Source: CAD feature listing. Evaluate the final solid. Frame: model axes, mm. Face numbers are marked on the shaded views. A direction names the side the tool comes from. Coordinates: 2 decimals unless noted, no trailing zeros. Order: outer loops, then holes, each group sorted by start corner. A loop starts at its lowest first (then second) coordinate and runs counter-clockwise, first axis right, second up.
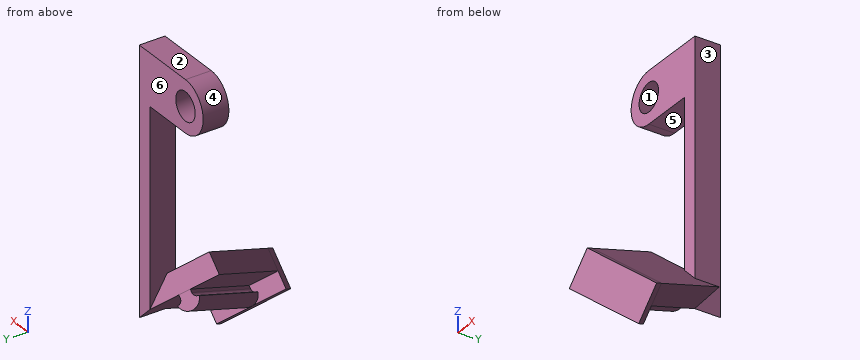
Autodesk Inventor part; units mm, degrees
ref_plane "YZ Plane" through (0, 0, 0) normal (1, 0, 0) x (0, 1, 0)
ref_plane "XZ Plane" through (0, 0, 0) normal (0, 1, 0) x (-1, 0, 0)
ref_plane "XY Plane" through (0, 0, 0) normal (0, 0, 1) x (1, 0, 0)
sketch "Sketch2" plane through (0, 0, 0) normal (0, 1, 0) x (-1, 0, 0)
  circle A0 centre (13.1, 80.1) radius 2.75
  circle A1 centre (80.1, 13.1) radius 2.75 construction
  line L0 (13.1, 80.1) -> (13.1, 13.1)
  line L1 (13.1, 13.1) -> (80.1, 13.1)
  line L2 (3, 37.224) -> (37.224, 3)
  line L3 (3, 37.224) -> (51.4, 37.224) construction
  circle A2 centre (80.1, 13.1) radius 2.75
  line L4 (3.1, 112.1) -> (3.1, 79.1)
  line L5 (79.1, 3.1) -> (112.1, 3.1)
  circle A3 centre (13.1, 80.1) radius 5
  line L6 (13.1, 75.1) -> (3, 75.1)
  line L7 (3, 75.1) -> (3, 3)
  line L8 (13.1, 85.1) -> (0, 85.1)
  line L9 (0, 85.1) -> (0, 0)
  circle A4 centre (80.1, 13.1) radius 5
  line L10 (85.1, 13.1) -> (85.1, 0)
  line L11 (75.1, 13.1) -> (75.1, 3)
  line L12 (75.1, 3) -> (3, 3)
  line L13 (85.1, 0) -> (0, 0)
  line L14 (3, 37.224) -> (-4.0711, 30.1529)
  line L15 (3, 37.224) -> (13, 37.224) construction
  point P0 (0, 0)
  point P1 (0, 34.224)
  dimension "d11" = 48.4
  dimension "d12" = 45
  dimension "d13" = 10
  dimension "d14" = 10.1
  dimension "d15" = 13.1
  dimension "d16" = 3
  dimension "d17" = 10
  dimension "d18" = 13.1
  dimension "d19" = 10.1
  dimension "d20" = 10
  dimension "d21" = 135
extrude "Extrusion2" add sketch "Sketch2" along normal blind 5 contours L6 L7 L14 L9 L8 A3 | A3
sketch "Sketch4" plane through (-3, 0, 37.224) normal (-0.7071068, 0, -0.7071068) x (-0.7071068, 0, 0.7071068)
  line L0 (0, 0) -> (0, 5)
  line L1 (0, 5) -> (-16.134, -14.2277)
  line L2 (0, 5) -> (25.1, 5) construction
  line L3 (-5.9456, -22.7768) -> (10.1884, -3.5491)
  line L4 (10.1884, -3.5491) -> (0, 5)
  line L5 (-5.9456, -22.7768) -> (-16.134, -14.2277)
  point P0 (-28.4426, 0)
  dimension "d33" = 130
  dimension "d34" = 25.1
  dimension "d35" = 13.3
  dimension "d37" = 25.1
extrude "Extrusion3" add sketch "Sketch4" against normal blind 4
sketch "Sketch6" plane through (0, -0.0562, 34.224) normal (-0.7071068, 0, -0.7071068) x (-0.7071068, 0, 0.7071068)
  line L0 (0, 5.0562) -> (4.2426, 5.0562)
  line L1 (0, 0.0562) -> (0, 5.0562)
  line L2 (0.0471, 0.0562) -> (-11.8913, -14.1715)
  line L3 (-11.8913, -14.1715) -> (-1.7029, -22.7206)
  line L4 (-1.7029, -22.7206) -> (14.431, -3.4929)
  line L5 (14.431, -3.4929) -> (4.2426, 5.0562)
  circle A0 centre (6.1229, -3.0486) radius 2.6
  line L6 (4.6432, 4.72) -> (14.755, -3.7647)
  circle A1 centre (-1.5906, -12.2411) radius 2.6
  line L7 (0, 0.0562) -> (0.0471, 0.0562)
  line L8 (14.431, -3.4929) -> (4.2426, 5.0562)
  line L9 (-6.7971, -18.4461) -> (10.7436, 2.4582)
  point P0 (-24.2, 0.0562)
  dimension "d38" = 5.2
  dimension "d39" = 5
  dimension "d40" = 12
extrude "Extrusion5" [suppressed]
fillet "Fillet1" [suppressed]
sketch "Sketch9" plane through (-0.1716, 0, 40.0524) normal (0.7071068, 0, 0.7071068) x (0.7071068, 0, -0.7071068)
  line L0 (4.1955, 0) -> (16.134, -14.2277)
  line L1 (16.134, -14.2277) -> (6.4922, -2.737)
  line L2 (6.4922, -2.737) -> (8.7903, -0.8087)
  line L3 (8.7903, -0.8087) -> (18.4321, -12.2994)
  line L4 (18.4321, -12.2994) -> (16.134, -14.2277)
  line L5 (5.9456, -22.7768) -> (16.134, -14.2277)
  line L6 (11.0398, -18.5023) -> (9.8066, -17.0326)
  line L7 (5.9456, -22.7768) -> (-3.6962, -11.2861)
  line L8 (-5.9944, -13.2145) -> (3.6474, -24.7052)
  line L9 (-3.6962, -11.2861) -> (-5.9944, -13.2145)
  line L10 (3.6474, -24.7052) -> (5.9456, -22.7768)
  point P0 (28.4426, 0)
  point P1 (4.6202, -0.5061)
  dimension "d46" = 15
  dimension "d47" = 3
extrude "Extrusion6" [suppressed]
sketch "Sketch10" plane through (8.4084, -14.2277, 25.8155) normal (0.4545195, -0.7660444, -0.4545195) x (0.7071068, 0, 0.7071068)
  line L0 (0, 0) -> (0, 13.3)
  line L1 (0, 0) -> (4, 0)
  line L2 (4, 13.3) -> (4, 0)
  line L3 (0, 13.3) -> (4, 13.3)
  line L4 (-0.6, 8.15) -> (0, 8.15)
  line L5 (0, -1.85) -> (0, 5.15)
  line L6 (0, 5.15) -> (-0.6, 5.15)
  arc A0 (-0.6, 5.15) -> (-1.099, 4.6815) centre (-0.6, 4.65) ccw
  arc A1 (-1.7225, 4.2287) -> (-1.099, 4.6815) centre (-1.598, 4.713) ccw
  arc A2 (-1.7225, 9.0713) -> (-1.7225, 4.2287) centre (-1.1, 6.65) ccw
  arc A3 (-1.099, 8.6185) -> (-1.7225, 9.0713) centre (-1.598, 8.587) ccw
  arc A4 (-1.099, 8.6185) -> (-0.6, 8.15) centre (-0.6, 8.65) ccw
  line L7 (0, 0) -> (0, 13.3)
  line L8 (0.6, 5.35) -> (-0.6, 5.35)
  arc A5 (-0.6, 5.35) -> (-1.2986, 4.6941) centre (-0.6, 4.65) ccw
  arc A6 (-1.6727, 4.4224) -> (-1.2986, 4.6941) centre (-1.598, 4.713) ccw
  arc A7 (-1.6727, 8.8776) -> (-1.6727, 4.4224) centre (-1.1, 6.65) ccw
  arc A8 (-1.2986, 8.6059) -> (-1.6727, 8.8776) centre (-1.598, 8.587) ccw
  arc A9 (-1.2986, 8.6059) -> (-0.6, 7.95) centre (-0.6, 8.65) ccw
  line L9 (-0.6, 7.95) -> (0.6, 7.95)
  line L10 (0.3, -1.85) -> (0.3, 5.45)
  line L11 (0.3, 5.45) -> (-0.6, 5.45)
  arc A10 (-0.6, 5.45) -> (-1.3984, 4.7004) centre (-0.6, 4.65) ccw
  arc A11 (-1.6478, 4.5193) -> (-1.3984, 4.7004) centre (-1.598, 4.713) ccw
  arc A12 (-1.6478, 8.7807) -> (-1.6478, 4.5193) centre (-1.1, 6.65) ccw
  arc A13 (-1.3984, 8.5996) -> (-1.6478, 8.7807) centre (-1.598, 8.587) ccw
  arc A14 (-1.3984, 8.5996) -> (-0.6, 7.85) centre (-0.6, 8.65) ccw
  line L12 (-0.6, 7.85) -> (0.4, 7.85)
  line L13 (0.4, -1.85) -> (0.4, 5.55)
  line L14 (0.4, 5.55) -> (-0.6, 5.55)
  arc A15 (-0.6, 5.55) -> (-1.4982, 4.7067) centre (-0.6, 4.65) ccw
  arc A16 (-1.6229, 4.6161) -> (-1.4982, 4.7067) centre (-1.598, 4.713) ccw
  arc A17 (-1.6229, 8.6839) -> (-1.6229, 4.6161) centre (-1.1, 6.65) ccw
  arc A18 (-1.4982, 8.5933) -> (-1.6229, 8.6839) centre (-1.598, 8.587) ccw
  arc A19 (-1.4982, 8.5933) -> (-0.6, 7.75) centre (-0.6, 8.65) ccw
  line L15 (-0.6, 7.75) -> (0.4, 7.75)
  point P0 (-24.2, -18.5744)
  point P1 (-11.4165, -11.1867)
  point P2 (0, 6.65)
  point P3 (0, 6.65)
  point P4 (0, 5.35)
  point P5 (0, 7.95)
  point P6 (0, 5.45)
  point P7 (0, 7.85)
  point P8 (0, 5.55)
  point P9 (0, 7.75)
  dimension "d64" = 2.5
  dimension "d65" = 0.6
  dimension "d66" = 1.1
  dimension "d67" = 0.2
  dimension "d68" = 0.3
  dimension "d69" = 0.4
extrude "Extrusion7" add sketch "Sketch10" against normal up to surface (25.1 mm away) contours L14 A15 A16 A17 A18 A19 L15 L0
sketch "Sketch11" plane through (11.2369, -14.2277, 28.644) normal (0.4545195, -0.7660444, -0.4545195) x (0.7071068, 0, 0.7071068)
  line L0 (-4, 0) -> (-4, 5.55)
  line L1 (-4, 0) -> (0, 0)
  line L2 (0, 13.3) -> (0, 0)
  line L3 (-4, 13.3) -> (0, 13.3)
  line L4 (0, 0) -> (0, 13.3)
  line L5 (0, 0) -> (-7.3, 0)
  line L6 (-7.7, 13.3) -> (0, 13.3)
  line L7 (0, 13.3) -> (0, 0)
  line L8 (-4, 7.75) -> (-4, 13.3)
  line L9 (-4, 7.75) -> (-4.6, 7.75)
  arc A0 (-5.4982, 8.5933) -> (-4.6, 7.75) centre (-4.6, 8.65) ccw
  arc A1 (-5.4982, 8.5933) -> (-5.6229, 8.6839) centre (-5.598, 8.587) ccw
  arc A2 (-5.6229, 8.6839) -> (-5.6229, 4.6161) centre (-5.1, 6.65) ccw
  arc A3 (-5.6229, 4.6161) -> (-5.4982, 4.7067) centre (-5.598, 4.713) ccw
  arc A4 (-4.6, 5.55) -> (-5.4982, 4.7067) centre (-4.6, 4.65) ccw
  line L10 (-4.6, 5.55) -> (-4, 5.55)
  line L11 (-7.2, 13.3) -> (-7.2, 0)
  arc A5 (-5.6229, 8.6839) -> (-5.6229, 4.6161) centre (-5.1, 6.65) ccw
  point P0 (-28.2, -18.5744)
  point P1 (-4, 0)
  point P2 (0, 13.3)
  point P3 (0, 0)
  point P4 (-4, 13.3)
  point P5 (-4, 13.3)
  point P6 (-4, 0)
  point P7 (-7.2, 6.65)
  point P8 (-7.2, 6.65)
extrude "Extrusion8" add sketch "Sketch11" along normal blind 2
properties part number "Pixy2 mount"
1. Ray query, line 1 (Z direction, x = -13.1, y = 4); line 2 (X direction, y = 3.55, z = 80.1); line 3 (Z direction, x = -3, y = -9). Return the intervals inside material, ascending.
Findings:
line 1: z = 75.1 to 77.35, 82.85 to 85.1
line 2: x = -18.1 to -15.85, -10.35 to 0
line 3: z = 32.7 to 35.45, 37.22 to 42.88
2. Section query C-C on y = -22. Return loops of the section in (x, z).
Findings:
outline: (-0.4, 30.1) - (1.8, 27.9) - (6.89, 32.99) - (3.57, 36.31) - (0.74, 33.48) - (1.86, 32.37) - close
3. Section query B-B on x = -11.5. Return loops of the section in (y, z), plus the area to 3 significant figures.
Findings:
outline: (0, 75.1) - (5, 75.1) - (5, 77.86) - (0, 77.86) - close; (0, 82.34) - (5, 82.34) - (5, 85.1) - (0, 85.1) - close
area: 27.6 mm2
4. Section query D-D on z = 52.5. Return loops of the section in (x, y).
Findings:
outline: (-3, 0) - (0, 0) - (0, 5) - (-3, 5) - close
5. Access query for the marked faces 5 and 6. Directions: +Z, -Z, +X, -X, +Y, -Y. A direction counts if a zero-diameter tool reaches every point of the face in a straight line with its end or side. Return the directions, or none.
Findings:
face 5: -X, +Y, -Y
face 6: +Z, -Z, +X, -X, +Y
6. Section query A-A on z = 80.1. Return loops of the section in (x, y), plus the area to 3 significant figures.
Findings:
outline: (-18.1, 0) - (-15.85, 0) - (-15.85, 5) - (-18.1, 5) - close; (-10.35, 0) - (0, 0) - (0, 5) - (-10.35, 5) - close
area: 63.0 mm2
7. Draft query along X for the marked faces 1, 2, 3 and 4. Return one class per face: released by +X, released by -X, zero draft, split by the parting line, or undercut.
Findings:
face 1: undercut
face 2: zero draft
face 3: released by +X
face 4: released by -X
8. Pin query (flat end, axial travel): P1, Ø1, axis at y = 2, z = 73, coming from the +X side; P2, Ø10, axis at x = -15, z = 71.5, coming from the -Y side; P3, Ø1.5, axis at y = 2.5, z = 64, coming from the -X side. Return the tip coordinate at first contact, or that it passes through.
Findings:
P1: stops at x = 0
P2: stops at y = 0
P3: stops at x = -3
